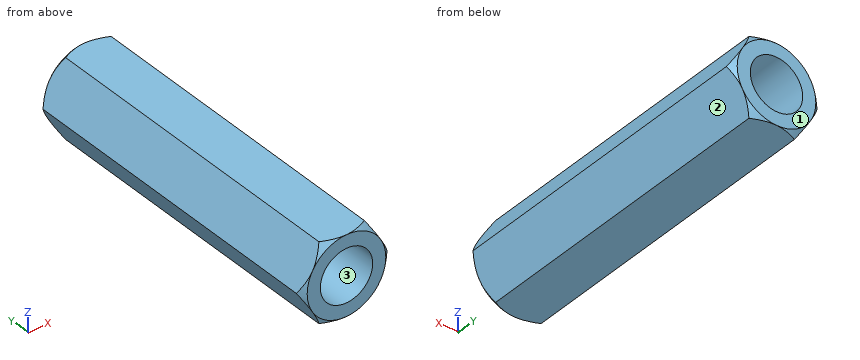
from build123d import *

# Parameters (mm, degrees)
SKETCH_1_R          = 3.5
SKETCH_1_R_2        = 2
EXTRUDE_1_DEPTH     = 25
CHAMFER_1_SIZE      = 0.5
SKETCH_2_OUTSIDE_W  = 14.378
SKETCH_2_OUTSIDE_H  = 14.378
CUT_EXTRUDE_1_DEPTH = 26


with BuildPart() as part:
    # 草图1 → 凸台-拉伸1 (new body)
    with BuildSketch(Plane(origin=(0, 0, 0), x_dir=(1, 0, 0), z_dir=(0, 1, 0))):
        Circle(SKETCH_1_R)
        Circle(SKETCH_1_R_2, mode=Mode.SUBTRACT)
    extrude(amount=EXTRUDE_1_DEPTH)

    # 倒角1
    chamfer_1_edges = [part.edges().sort_by_distance(p)[0] for p in [
        (-3.5, 0, 0),
        (-3.5, 25, 0),
    ]]
    chamfer(chamfer_1_edges, length=CHAMFER_1_SIZE)

    # 草图2 outside → 切除-拉伸1 (cut, through all)
    with BuildSketch(Plane(origin=(0, 25, 0), x_dir=(1, 0, 0), z_dir=(0, 1, 0))):
        Rectangle(SKETCH_2_OUTSIDE_W, SKETCH_2_OUTSIDE_H)
        Polygon((1.732050808, 3), (-1.732050808, 3), (-3.464101615, 0), (-1.732050808, -3), (1.732050808, -3), (3.464101615, 0), align=None, mode=Mode.SUBTRACT)
    extrude(amount=-CUT_EXTRUDE_1_DEPTH, mode=Mode.SUBTRACT)


solid = part.part
Design review of the part built by this model. Coordinates are the model's own, in mm. Face numbers are marked on the shaded views. Round coordinates to 2 decimals unless told otherwise and drop trailing zeros. Write each loop counter-clockwise with the first axis right and the second up, starting at its lowest first coordinate (ties: lowest second). Pieces come first, ordered by that corner, then holes. Notation, with made-up numbers: (-4.75, -37) -> (5.25, -37) arc R14 ccw to (5.25, -12) -> close; hole circle Ø11 at (63, 71.25). An arc over 180 degrees is marked (long way). One line per item, written item: value. Start each with the question number.
Q1. Add section A-A (y = 16.25). Give the boundary of the cut face in (x, z).
Q2. Insertion check: P1, Ø1.5, axis at y = 3.5, z = -2, coming from the -X side; P2, Ø1.5, axis at y = 22, z = -1, coming from the -X side. Each pin has a flat end and moves straight along its axis. Give the tip position at first contact, or say it passes through.
Q3. To check wall thickness, follow probe 1 along Z at (x, y) = (-1, 8.75); probe 2 along Z at (x, y) = (0, 10.25); probe 3 along X at (y, z) = (19, -0.5). State the ranges of each line that lie inside material, in increasing order.
Q4. The part is to be moulded in two halves that separate along Z. For the marked faces 1, 2 and 3, say which applies: pulls with the +Z half, pulls with the -Z half, needs draft (parallel to the pull), parting line crosses it, or undercut.
Response:
1. outline: (-3.46, 0) -> (-1.73, -3) -> (1.73, -3) -> (3.46, 0) -> (1.73, 3) -> (-1.73, 3) -> close; hole circle Ø4 at (0, 0)
2. P1: stops at x = -2.74
2. P2: stops at x = -3.32
3. probe 1: z = -3 to -1.73, 1.73 to 3
3. probe 2: z = -3 to -2, 2 to 3
3. probe 3: x = -3.18 to -1.94, 1.94 to 3.18
4. face 1: needs draft
4. face 2: pulls with the -Z half
4. face 3: undercut
